Read the model definition and answer for the solid it produces. Units are mm, in the model's axes. A direction names the side the tool comes from. Coordinates: 2 decimals unless noted, no trailing zeros. Order: outer loops, then holes, each group sorted by start corner. A loop starts at its lowest first (then second) coordinate and runs counter-clockwise, first axis right, second up. Notation, with made-up numbers: (42.5, -36) - (97.5, -36) arc R26 cw to (97.5, -7) - close; hole circle Ø8 at (-25.75, -8.5). An arc over 180 degrees is marked (long way). Write item = value, one per line.
from build123d import *

# Parameters (mm, degrees)
SKETCH_1_R          = 3.25
EXTRUDE_1_DEPTH     = 22
SKETCH_2_R          = 4.85
CUT_EXTRUDE_3_DEPTH = 20
SKETCH_3_R          = 6
CUT_EXTRUDE_4_DEPTH = 18


with BuildPart() as part:
    # 草图1 → 凸台-拉伸1 (new body)
    with BuildSketch(Plane(origin=(0, 0, 0), x_dir=(1, 0, 0), z_dir=(0, 1, 0))):
        Polygon((-28.8, 26.85), (-23.8, 31.85), (23.8, 31.85), (28.8, 26.85), (28.8, -26.85), (23.8, -31.85), (-23.8, -31.85), (-28.8, -26.85), align=None)
        with Locations(Location((2.5, 27, 0), (0, 0, 270))):
            Circle(SKETCH_1_R, mode=Mode.SUBTRACT)
        with Locations(Location((2.5, -27, 0), (0, 0, 90))):
            Circle(SKETCH_1_R, mode=Mode.SUBTRACT)
    extrude(amount=EXTRUDE_1_DEPTH)

    # 草图2 → 切除-拉伸3 (cut)
    # profile 1 of 2: a face of its own
    with BuildSketch(Plane(origin=(0, 22, 0), x_dir=(1, 0, 0), z_dir=(0, 1, 0))):
        Polygon((-10, -19.891494973), (10, -19.891494973), (10, -31.85), (10, -34.308434643), (-10, -34.308434643), (-10, -31.85), align=None)
        with Locations(Location((2.5, -27, 0), (0, 0, 270))):
            Circle(SKETCH_2_R, mode=Mode.SUBTRACT)
    # profile 2 of 2: a face of its own
    with BuildSketch(Plane(origin=(0, 22, 0), x_dir=(1, 0, 0), z_dir=(0, 1, 0))):
        Polygon((-10, 19.891494973), (-10, 31.85), (-10, 34.247261474), (10, 34.247261474), (10, 31.85), (10, 19.891494973), align=None)
        with Locations(Location((2.5, 27, 0), (0, 0, 270))):
            Circle(SKETCH_2_R, mode=Mode.SUBTRACT)
    extrude(amount=-CUT_EXTRUDE_3_DEPTH, mode=Mode.SUBTRACT)

    # 草图3 → 切除-拉伸4 (cut)
    with BuildSketch(Plane(origin=(0, 22, 0), x_dir=(1, 0, 0), z_dir=(0, 1, 0))):
        with Locations((2.5, 27)):
            Circle(SKETCH_3_R)
        with Locations((2.5, -27)):
            Circle(SKETCH_3_R)
    extrude(amount=-CUT_EXTRUDE_4_DEPTH, mode=Mode.SUBTRACT)


solid = part.part
1) The part is cut by section B-B (y = 12). Determine the outline of the cut face in (x, z), and give its area (3 significant figures).
Returned:
outline = (-28.8, -26.85) - (-23.8, -31.85) - (-10, -31.85) - (-10, -19.89) - (10, -19.89) - (10, -31.85) - (23.8, -31.85) - (28.8, -26.85) - (28.8, 26.85) - (23.8, 31.85) - (10, 31.85) - (10, 19.89) - (-10, 19.89) - (-10, 31.85) - (-23.8, 31.85) - (-28.8, 26.85) - close
area = 3,140 mm^2
2) The part is cut by section A-A (y = 2.75). Determine the outline of the cut face in (x, z).
Returned:
outline = (-28.8, -26.85) - (-23.8, -31.85) - (-10, -31.85) - (-10, -19.89) - (10, -19.89) - (10, -31.85) - (23.8, -31.85) - (28.8, -26.85) - (28.8, 26.85) - (23.8, 31.85) - (10, 31.85) - (10, 19.89) - (-10, 19.89) - (-10, 31.85) - (-23.8, 31.85) - (-28.8, 26.85) - close; circle Ø9.7 at (2.5, -27); circle Ø9.7 at (2.5, 27); hole circle Ø6.5 at (2.5, -27); hole circle Ø6.5 at (2.5, 27)
3) Straight lines are drawn through the part: line 1 along X through (y, z) = (18.25, 22.5); line 2 along Y through (x, z) = (7.5, -28); line 3 along X through (y, z) = (1, 27). For each, find the intervals that lie inside material, in ascending order. Write a range as from..to.
Returned:
line_1 = -28.8..-10, 10..28.8
line_2 = 0..2
line_3 = -28.65..-0.75, 5.75..28.65
4) Determine the mould class of faces 1 (the face through (0, 22, 0)), 2 (the face through (-2, 2, 24)), 3 (the face through (-26.335, 10.846, -29.315)) for opening direction X: pulls with the +X half, pulls with the -X half, needs draft (parallel to the pull), parting line crosses it, or undercut.
Returned:
face_1 = needs draft
face_2 = undercut
face_3 = pulls with the -X half
5) Flat-ended cylindrical pins translate along their axes: pin 1 Ø6 at (x, z) = (2.5, 27) entering from -Y; pin 2 Ø3.5 at (x, z) = (0.5, 26) entering from +Y; pin 3 Ø2 at (x, y) = (7, 10) entering from +Z. Find the tip coordinate at first contact, or state that the pin passes through.
Returned:
pin_1 = through
pin_2 = 4
pin_3 = 19.89
6) For faces 4 (the face through (10, 12, 26)), 5 (the face through (26.265, 10.846, -29.385)), 6 (the face through (2.713, 3.014, 22.155)), determine the directions among +Z, -Z, +X, -X, +Y, -Y from which every point of the face is accessible in a straight line to the end or side of a thin tool.
Returned:
face_4 = +Z, +Y
face_5 = -Z, +X, +Y, -Y
face_6 = +Y
